The listing builds one solid part. Answer for the finished solid, in the listing's coordinates (mm). Coordinates: 2 decimals unless noted, no trailing zeros. Loops run counter-clockwise (first coordinate to the right, second up) from the corner with the lowest first, then second, coordinate; pieces in that order, holes last. Notation, with made-up numbers: (4, -21.5) - (52, -21.5) arc R16 ccw to (52, -2.5) - close; hole circle Ø3 at (66.25, 12). An arc over 180 degrees is marked (long way). Return JSON: item names as keys, results as strings. Group by question number.
1. Find the intervals of material crossed by line 1 along Y through (x, z) = (11, 1.9); line 2 along Y through (x, z) = (8, 0.75); line 3 along X through (y, z) = (19, 1.9), in increasing order.
2. Section B-B (z = 1.35) is taken. Write down the section's boundary in (x, y), and give its area (3 significant figures).
3. Each of these flat-tipped pins is pushed along its axis until it touches: P1, Ø6, axis at x = 17, y = 15.5, coming from the -Z side; P2, Ø4, axis at x = 9.906, y = 12.7, coming from the +Z side. Where does it stop, or does it pass through?
4. The mould has two halves that part along Y. Classify faces 1 (the face through (12, 20.32, 1)), 2 (the face through (11.681, 15.484, 1.252)), 3 (the face through (10, 0, 1)), 4 (the face through (10, 8, 2.54)): pulls with the +Y half, pulls with the -Y half, needs draft (parallel to the pull), parting line crosses it, or undercut.
5. Section A-A (y = 12.7) is taken. Write down the section's boundary in (x, z), and give its area (3 significant figures).
6. Section C-C (y = 14.75) is taken. Write down the section's boundary in (x, z), and give its area (3 significant figures).
```python
from build123d import *

# Parameters (mm, degrees)
SKETCH1_R           = 3.302
BOSS_EXTRUDE1_DEPTH = 2.54


with BuildPart() as part:
    # Sketch1 → Boss-Extrude1 (new body)
    with BuildSketch(Plane.XY):
        Polygon((0, 15.24), (5.08, 20.32), (19.812, 20.32), (19.812, 0), (0, 0), align=None)
        with Locations((9.906, 12.7)):
            Circle(SKETCH1_R, mode=Mode.SUBTRACT)
    extrude(amount=BOSS_EXTRUDE1_DEPTH)


solid = part.part
```
The answers:
{
 "1": {"line 1": "y = 0 to 9.58, 15.82 to 20.32", "line 2": "y = 0 to 10, 15.4 to 20.32", "line 3": "x = 3.76 to 19.81"},
 "2": {"outline": "(0, 0) - (19.81, 0) - (19.81, 20.32) - (5.08, 20.32) - (0, 15.24) - close; hole circle Ø6.6 at (9.91, 12.7)", "area": "355 mm2"},
 "3": {"P1": "stops at z = 0", "P2": "passes through"},
 "4": {"face 1": "pulls with the +Y half", "face 2": "undercut", "face 3": "pulls with the -Y half", "face 4": "needs draft"},
 "5": {"outline": "(0, 0) - (6.6, 0) - (6.6, 2.54) - (0, 2.54) - close; (13.21, 0) - (19.81, 0) - (19.81, 2.54) - (13.21, 2.54) - close", "area": "33.5 mm2"},
 "6": {"outline": "(0, 0) - (7.32, 0) - (7.32, 2.54) - (0, 2.54) - close; (12.49, 0) - (19.81, 0) - (19.81, 2.54) - (12.49, 2.54) - close", "area": "37.2 mm2"}
}
